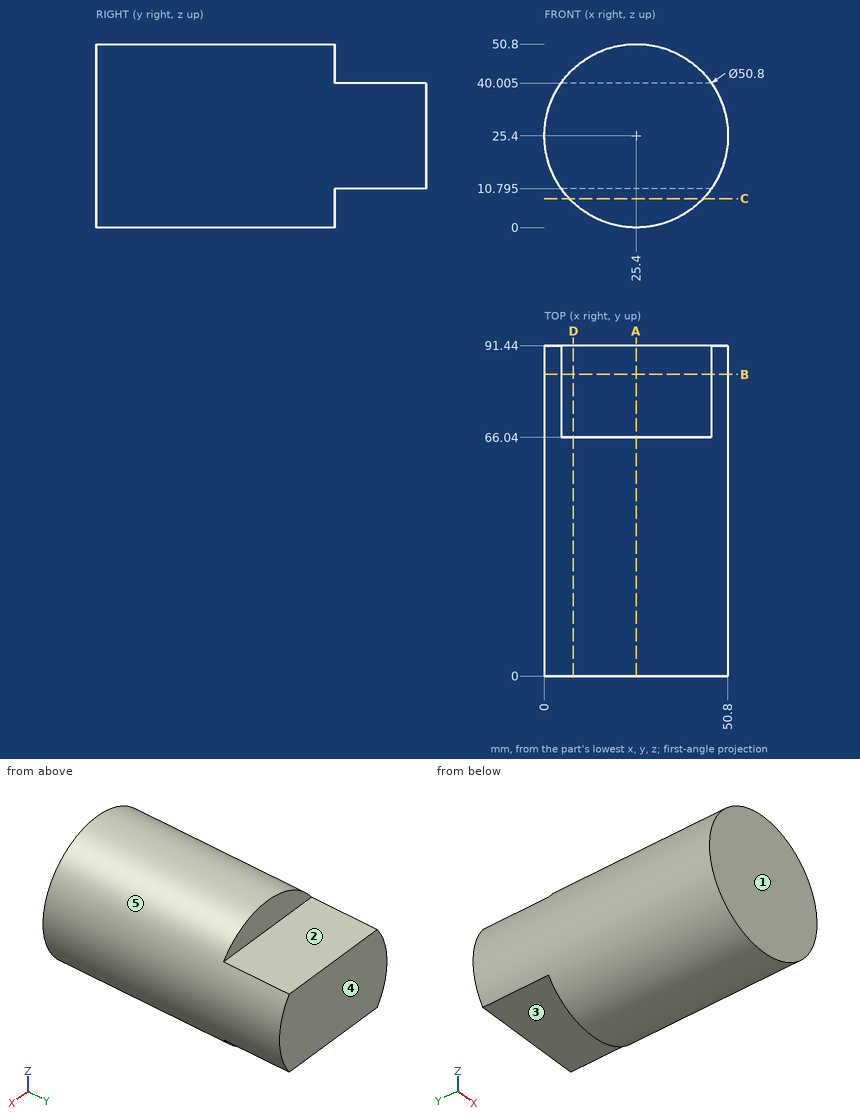
Check sheet for the drawn part. Datum: minimum x, y, z corner. Units: mm. A direction names the side the tool comes from. Give positions to 0.01 mm unless a question says otherwise; leave off trailing zeros. Loops run counter-clockwise (first coordinate to the right, second up) from the corner with the lowest first, then second, coordinate; pieces in that order, holes last.
1) Draft check along Z on the marked faces 3, 4 and 5. Enter one of: pulls with the +Z half, pulls with the -Z half, needs draft (parallel to the pull), parting line crosses it, or undercut.
2) Sectioned sample at C-C, the plane z = 8. Enter the section's corners in (x, y), then the cut area to 3 significant figures.
3) Set-up check for the marked faces 1 and 2: record each of +Z, -Z, +X, -X, +Y, -Y from which the full face is reachable in a straight line by a thin tool's end or side.
4) Thickness scan on line 1 along Y through (x, z) = (21.5, 48.5); line 2 along Z through (x, y) = (20.5, 81.5) (3 decimals); line 3 along X through (y, z) = (31, 45). Record the ranges inside material, lowest first.
5) Sectioned sample at B-B, the plane y = 83.5. Enter the section's corners in (x, z) (3 decimals).
6) Sectioned sample at D-D, the plane x = 8. Enter the section's corners in (y, z) (3 decimals).
7) Sectioned sample at A-A, the plane x = 25.4. Enter the section's corners in (y, z) (3 decimals), then the cut area to 3 significant figures.
8) Depth check by flat-ended pin: pin 1 Ø1 at (x, y) = (12, 39.5) entering from +Z; pin 2 Ø4 at (y, z) = (12, 13) entering from -X; pin 3 Ø3 at (x, z) = (31, 5) entering from +Y. Enter the tip coordinate at first touch or a pass-through.
Answers:
1. face 3: pulls with the -Z half
1. face 4: needs draft
1. face 5: parting line crosses it
2. outline: (6.9, 0) - (43.9, 0) - (43.9, 66.04) - (6.9, 66.04) - close
2. area: 2,440 mm2
3. face 1: +Z, -Z, +X, -X, -Y
3. face 2: +Z, +X, -X, +Y
4. line 1: y = 0 to 66.04
4. line 2: z = 10.795 to 40.005
4. line 3: x = 9.24 to 41.56
5. outline: (4.619, 10.795) - (46.181, 10.795) arc R25.4 ccw to (46.181, 40.005) - (4.619, 40.005) arc R25.4 ccw to start
6. outline: (0, 6.896) - (66.04, 6.896) - (66.04, 10.795) - (91.44, 10.795) - (91.44, 40.005) - (66.04, 40.005) - (66.04, 43.904) - (0, 43.904) - close
7. outline: (0, 0) - (66.04, 0) - (66.04, 10.795) - (91.44, 10.795) - (91.44, 40.005) - (66.04, 40.005) - (66.04, 50.8) - (0, 50.8) - close
7. area: 4,100 mm2
8. pin 1: stops at z = 47.28
8. pin 2: stops at x = 2.23
8. pin 3: stops at y = 66.04
